Model file for the job. Use its own axes, mm. A direction names the side the tool comes from. Coordinates: 2 decimals unless noted, no trailing zeros. Order: outer loops, then holes, each group sorted by start corner. A loop starts at its lowest first (then second) coordinate and runs counter-clockwise, first axis right, second up.
from build123d import *

# Parameters (mm, degrees)
SKIZZE1_R                       = 30
AUFSATZ_LINEAR_AUSTRAGEN1_DEPTH = 32
SKIZZE2_R                       = 14.996636578
AUFSATZ_LINEAR_AUSTRAGEN2_DEPTH = 2
SKIZZE3_R                       = 4.75
AUFSATZ_LINEAR_AUSTRAGEN3_DEPTH = 10
SKIZZE4_R                       = 4
SCHNITT_LINEAR_AUSTRAGEN1_DEPTH = 10


with BuildPart() as part:
    # Skizze1 → Aufsatz-Linear austragen1 (new body)
    with BuildSketch(Plane.XY):
        Circle(SKIZZE1_R)
    extrude(amount=AUFSATZ_LINEAR_AUSTRAGEN1_DEPTH)

    # Skizze2 → Aufsatz-Linear austragen2 (add)
    with BuildSketch(Plane(origin=(0, 0, 0), x_dir=(-1, 0, 0), z_dir=(0, 0, -1))):
        Circle(SKIZZE2_R)
    extrude(amount=AUFSATZ_LINEAR_AUSTRAGEN2_DEPTH)

    # Skizze3 → Aufsatz-Linear austragen3 (add)
    with BuildSketch(Plane(origin=(0, 0, -2), x_dir=(-1, 0, 0), z_dir=(0, 0, -1))):
        Circle(SKIZZE3_R)
    extrude(amount=AUFSATZ_LINEAR_AUSTRAGEN3_DEPTH)

    # Skizze4 → Schnitt-Linear austragen1 (cut)
    with BuildSketch(Plane(origin=(0, 0, -12), x_dir=(-1, 0, 0), z_dir=(0, 0, -1))):
        Circle(SKIZZE4_R)
    extrude(amount=-SCHNITT_LINEAR_AUSTRAGEN1_DEPTH, mode=Mode.SUBTRACT)


solid = part.part
Q1. Which spindle directions (+Z, -Z, +X, -X, +Y, -Y) get a long thin tool onto all of the face, cutting with end or side? Do faces 4 (the face through (6, 14, 0)), 5 (the face through (0, 0, 32)). Say none if no direction does.
Established:
face 4: -Z
face 5: +Z, +X, -X, +Y, -Y
Q2. Cut at C-C, the plane z = 4. List the corners of the cut face in (x, y), plus the area to 3 significant figures.
Established:
outline: circle Ø60 at (0, 0)
area: 2,830 mm2
Q3. Mould opens along Y. For faces 1 (the face through (-2.192, -4.214, -6.93)), 2 (the face through (0, 0, -2)), 3 (the face through (4, 4, -2)) say: pulls with the +Y half, pulls with the -Y half, needs draft (parallel to the pull), parting line crosses it, or undercut.
Established:
face 1: parting line crosses it
face 2: undercut
face 3: needs draft
Q4. Cut at D-D, the plane z = -4.5. List the corners of the cut face in (x, y).
Established:
outline: circle Ø9.5 at (0, 0); hole circle Ø8 at (0, 0)
Q5. Cut at A-A, the plane y = 0. List the corners of the cut face in (x, z), plus the area to 3 significant figures.
Established:
outline: (-30, 0) - (-15, 0) - (-15, -2) - (-4.75, -2) - (-4.75, -12) - (-4, -12) - (-4, -2) - (4, -2) - (4, -12) - (4.75, -12) - (4.75, -2) - (15, -2) - (15, 0) - (30, 0) - (30, 32) - (-30, 32) - close
area: 1,990 mm2
Q6. Drop flat-ended pins along their axis: P1, Ø2, axis at y = -4, z = -6, coming from the -X side; P2, Ø6, axis at y = 23.5, z = 16, coming from the +X side; P3, Ø3, axis at y = -14, z = 0.5, coming from the +X side; P4, Ø9, axis at x = -0.5, y = -1.5, coming from the -Z side. Give the stop position or say it passes through.
Established:
P1: stops at x = -3.68
P2: stops at x = 21.9
P3: stops at x = 27.27
P4: stops at z = -12
Q7. Probe line 1 (Y direction, x = 0, z = -6); line 2 (Z direction, x = -27, y = 8); line 3 (X direction, y = 1, z = 16). List the from-to ranges inside material, lowest first.
Established:
line 1: y = -4.75 to -4, 4 to 4.75
line 2: z = 0 to 32
line 3: x = -29.98 to 29.98
